Build history of the part. All positions in model axes, mm. A direction names the side the tool comes from. Give positions to 0.01 mm unless a question says otherwise; leave off trailing zeros. Order: outer loops, then holes, each group sorted by start corner. A loop starts at its lowest first (then second) coordinate and runs counter-clockwise, first axis right, second up. Notation, with made-up numbers: M 85,13 L 93,13 A20 ccw 93,40 Z; hole C 6,9.25 d8. An arc over 180 degrees is marked long. Answer as CSV lines item,"result".
Autodesk Inventor part; units mm, degrees
ref_plane "YZ Plane" through (0, 0, 0) normal (1, 0, 0) x (0, 1, 0)
ref_plane "XZ Plane" through (0, 0, 0) normal (0, 1, 0) x (-1, 0, 0)
ref_plane "XY Plane" through (0, 0, 0) normal (0, 0, 1) x (1, 0, 0)
sketch "Sketch5" plane through (0, 0, 0) normal (0, 0, 1) x (1, 0, 0)
  line L0 (52.8, -15.6) -> (52.8, -10.6)
  line L1 (52.8, -10.6) -> (49.8, -10.6)
  line L2 (49.8, -10.6) -> (49.8, -12.55)
  line L3 (44, -12.55) -> (44, -3.05)
  line L4 (49.8, -3.05) -> (49.8, -5)
  line L5 (49.8, -5) -> (52.8, -5)
  line L6 (52.8, -5) -> (52.8, 0)
  line L7 (52.8, 0) -> (7.8, 0)
  line L8 (44, -3.05) -> (49.8, -3.05)
  line L9 (44, -12.55) -> (49.8, -12.55)
  line L10 (52.8, -15.6) -> (7.8, -15.6)
  arc A0 (7.8, 0) -> (7.8, -15.6) centre (7.8, -7.8) ccw
  point P0 (0, 0)
  dimension "d41" = 5.8
  dimension "d48" = 44
  dimension "d50" = 3
  dimension "d63" = 45
  dimension "d67" = 15.6
  dimension "d71" = 0
  dimension "d72" = 36.2
  dimension "d80" = 5.6
  dimension "d81" = 9.5
extrude "Extrusion2" add sketch "Sketch5" along normal blind 12
sketch "Sketch7" plane through (0, 0, 12) normal (0, 0, 1) x (1, 0, 0)
  line L0 (52.8, 0) -> (7.8, 0)
  line L1 (7.8, 0) -> (0, 0)
  line L2 (0, 0) -> (0, -15.6)
  line L3 (0, -15.6) -> (7.8, -15.6)
  line L4 (7.8, -15.6) -> (7.8, 0)
  point P0 (0, 0)
extrude "Extrusion4" cut sketch "Sketch7" against normal through all
sketch "Sketch9" plane through (0, 0, 12) normal (0, 0, 1) x (1, 0, 0)
  line L0 (52.8, 0) -> (7.8, 0)
  line L1 (7.8, 0) -> (-6.2954, -5.1303)
  line L2 (-6.2954, -5.1303) -> (-0.9599, -19.7895)
  line L3 (-0.9599, -19.7895) -> (13.1355, -14.6592)
  line L4 (7.8, 0) -> (13.1355, -14.6592)
  line L5 (7.8, 0) -> (7.8, -15.6)
  point P0 (0, 0)
  dimension "d83" = 15.6
  dimension "d84" = 20
  dimension "d85" = 90
  dimension "d86" = 20
  dimension "d87" = 15
  dimension "d90" = 15
extrude "Extrusion5" add sketch "Sketch9" against normal up to surface (12 mm away)
equation "\"l1\" = 8"
properties part number "Finray_test_8_Flach_winkel10deg"
Item 1: Band-saw the part on C-C (z = 2.25). Give the cut face in (x, y), and give its area (3 significant figures).
Geometry says:
outline,"M -6.3,-5.13 L -0.96,-19.79 L 10.55,-15.6 L 52.8,-15.6 L 52.8,-10.6 L 49.8,-10.6 L 49.8,-12.55 L 44,-12.55 L 44,-3.05 L 49.8,-3.05 L 49.8,-5 L 52.8,-5 L 52.8,0 L 7.8,0 Z"
area,"821 mm2"
Item 2: Band-saw the part on A-A (x = 45). Give the cut face in (y, z), and give its area (3 significant figures).
Geometry says:
outline,"M -15.6,0 L -12.55,0 L -12.55,12 L -15.6,12 Z; M -3.05,0 L 0,0 L 0,12 L -3.05,12 Z"
area,"73.2 mm2"
Item 3: 3-axis set-ups, long thin cutter, end or side, ignore diameter. For faces 5 (the flat face through (32, -15.6, 6)), 6 (the flat face through (-3.665, -12.357, 6.084)), 7 (the flat face through (51, -10.6, 6)), 8 (the flat face through (23, -8, 12)), 9 (the flat face through (44, -8, 6)): which of +Z, -Z, +X, -X, +Y, -Y reach the whole face in a straight line?
Geometry says:
face 5,"+Z, -Z, +X, -Y"
face 6,"+Z, -Z, -X, -Y"
face 7,"+Z, -Z, +X"
face 8,"+Z, +X, -X, +Y, -Y"
face 9,"+Z, -Z"
Item 4: Band-saw the part on B-B (y = -11.75). Give the cut face in (x, z).
Geometry says:
outline,"M -3.89,0 L 44,0 L 44,12 L -3.89,12 Z; M 49.8,0 L 52.8,0 L 52.8,12 L 49.8,12 Z"
Item 5: Probe line 1 along Y through (x, z) = (47.5, 9.25); line 2 along Y through (x, z) = (25.5, 5.5); line 3 along X through (y, z) = (-14.25, 9). List the from-to ranges inside material, lowest first. Write a range as from..to.
Geometry says:
line 1,"y = -15.6..-12.55, -3.05..0"
line 2,"y = -15.6..0"
line 3,"x = -2.98..52.8"
Item 6: Pull direction Y, two halves, no side cores. Call faces 1 (the flat face through (0.85, -2.53, 6.08)), 2 (the flat face through (47, -3.05, 6)), 3 (the flat face through (4.715, -17.724, 6.084)), 4 (the flat face through (49.8, -12, 6)): released by +Y, released by -Y, zero draft, split by the parting line, or undercut.
Geometry says:
face 1,"released by +Y"
face 2,"undercut"
face 3,"released by -Y"
face 4,"undercut"
Item 7: Drop flat-ended pins along their axis: pin 1 (3 mm diameter, centred on y = -7, z = 8, fed in from +X); pin 2 (1.6 mm diameter, centred on y = -11.5, z = 7, fed in from -X); pin 3 (1.5 mm diameter, centred on y = -17, z = 1.5, fed in from -X). Give the stop position or say it passes through.
Geometry says:
pin 1,"stops at x = 44"
pin 2,"stops at x = -4.27"
pin 3,"stops at x = -2.25"
Item 8: Band-saw the part on D-D (y = -17). Give the cut face in (x, z), and give its area (3 significant figures).
Geometry says:
outline,"M -1.98,0 L 6.7,0 L 6.7,12 L -1.98,12 Z"
area,"104 mm2"
